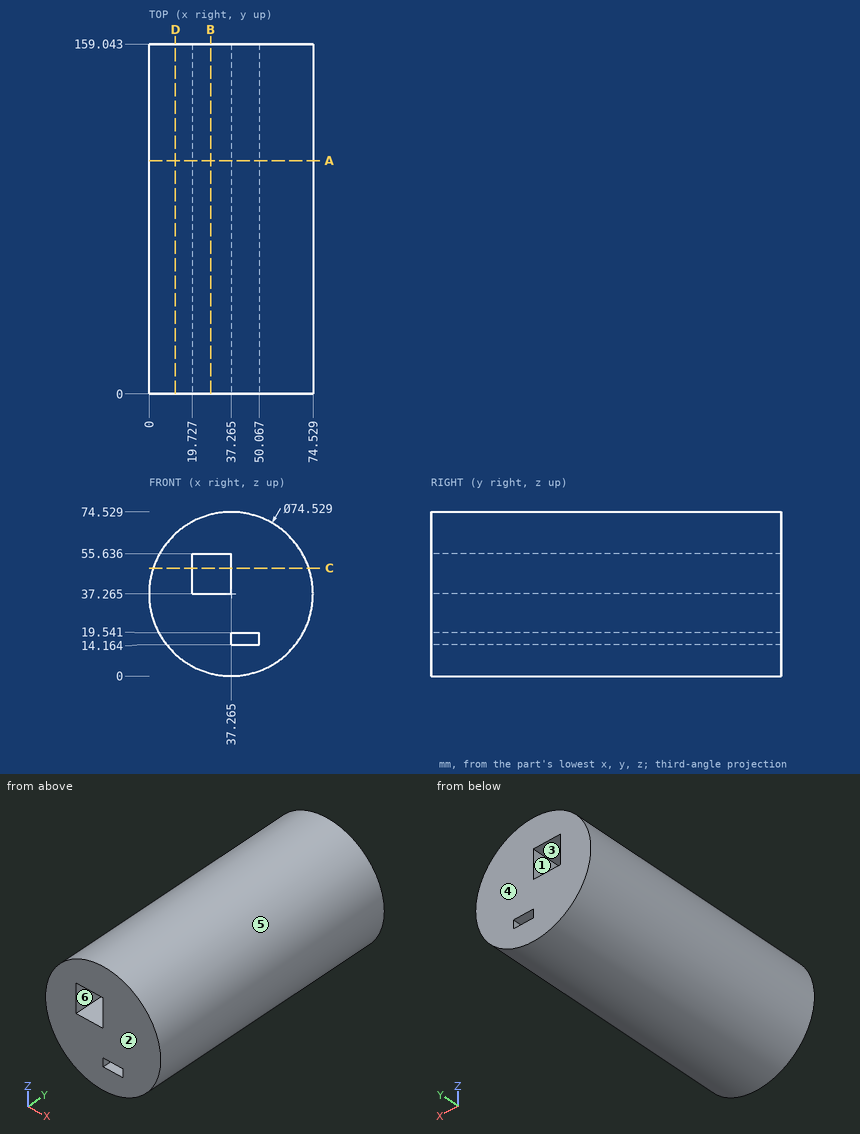
Input: dimensioned drawing with shaded views. Units: mm. Origin: part minimum x, y, z. A direction names the side the tool comes from. Round coordinates to 2 decimals unless told otherwise and drop trailing zeros. Loops run counter-clockwise (first coordinate to the right, second up) from the corner with the lowest first, then second, coordinate; pieces in that order, holes last. Notation, with made-up numbers: (58.5, 73.25) -> (62.5, 73.25) arc R15 cw to (62.5, 88.25) -> close; hole circle Ø6 at (20, -8.5). An arc over 180 degrees is marked (long way). One line per item, written item: value.
(1) Material intervals for line 1 (X direction, y = 30, z = 15.5) (1 decimal); line 2 (Z direction, x = 33.5, y = 134.5) (1 decimal); line 3 (Z direction, x = 46, y = 123) (1 decimal), sorted ascending. Write a range as [from, to].
Geometry check:
line 1: [7, 37.3], [50.1, 67.5]
line 2: [0.2, 37.3], [55.6, 74.3]
line 3: [1, 14.2], [19.5, 73.5]
(2) Section A-A (y = 106). Return the cut outline in (x, z) (1 decimal), plus the area to 3 significant figures.
Geometry check:
outline: circle Ø74.5 at (37.3, 37.3); hole (19.7, 37.3) -> (37.3, 37.3) -> (37.3, 55.6) -> (19.7, 55.6) -> close; hole (37.3, 14.2) -> (50.1, 14.2) -> (50.1, 19.5) -> (37.3, 19.5) -> close
area: 3,970 mm2
(3) Section B-B (x = 28). Return the cut outline in (y, z) (1 decimal), plus the area to 3 significant figures.
Geometry check:
outline: (0, 1.2) -> (159, 1.2) -> (159, 37.3) -> (0, 37.3) -> close; (0, 55.6) -> (159, 55.6) -> (159, 73.4) -> (0, 73.4) -> close
area: 8,560 mm2
(4) Set-up query: the marked faces 1 and 2. Return all of +Z, -Z, +X, -X, +Y, -Y with unobstructed straight access to the full face (end or side cutting, diameter ignored); none if empty.
Geometry check:
face 1: +Y, -Y
face 2: +Z, -Z, +X, -X, -Y
(5) Pin query (flat end, axial travel): pin 1 (1 mm diameter, centred on x = 8, y = 40.5, fed in from +Z) (1 decimal); pin 2 (19.5 mm diameter, centred on x = 26, y = 105.5, fed in from +Z); pin 3 (12 mm diameter, centred on x = 32.5, y = 138, fed in from -Z); pin 4 (6 mm diameter, centred on y = 32.5, z = 38, fed in from -X). Return the tip coordinate at first contact, or that it passes through.
Geometry check:
pin 1: z = 61
pin 2: z = 74.5
pin 3: z = 0
pin 4: x = 0
(6) Section C-C (z = 49). Return the cut outline in (x, y) (1 decimal).
Geometry check:
outline: (1.9, 0) -> (19.7, 0) -> (19.7, 159) -> (1.9, 159) -> close; (37.3, 0) -> (72.6, 0) -> (72.6, 159) -> (37.3, 159) -> close
(7) Mould query, pull axis X, two halves, no side actions, for the marked faces 3, 4, 5 and 6. Classes: pulls with the +X half, pulls with the -X half, needs draft (parallel to the pull), parting line crosses it, or undercut.
Geometry check:
face 3: undercut
face 4: needs draft
face 5: parting line crosses it
face 6: undercut
(8) Section D-D (x = 12). Return the cut outline in (y, z).
Geometry check:
outline: (0, 9.87) -> (159.04, 9.87) -> (159.04, 64.66) -> (0, 64.66) -> close
